from build123d import *

# Parameters (mm, degrees)
SKETCH_1_W           = 53
SKETCH_1_H           = 35
EXTRUDE_1_DEPTH      = 3.92
SKETCH_2_W           = 12
SKETCH_2_H           = 27
CUT_EXTRUDE_1_DEPTH  = 4
EXTRUDE_2_DEPTH      = 16.08
EXTRUDE_2_DEPTH_BACK = 3.92
SKETCH_3_W           = 12
SKETCH_3_H           = 7
SKETCH_4_W           = 12
SKETCH_4_H           = 3.92
EXTRUDE_3_DEPTH      = 8
SKETCH_5_R           = 2.86
CUT_EXTRUDE_2_DEPTH  = 37.889245045
EXTRUDE_4_DEPTH      = 4
SKETCH_8_W           = 53
SKETCH_8_H           = 3.92
EXTRUDE_5_DEPTH      = 20
FILLET_1_R           = 2.5
FILLET_2_R           = 11
FILLET_3_R           = 1
FILLET_4_R           = 2
SKETCH_9_W           = 20.08
SKETCH_9_H           = 8
CUT_EXTRUDE_5_DEPTH  = 67.886593574
SKETCH_6_R           = 6
CUT_EXTRUDE_3_DEPTH  = 6.5


with BuildPart() as part:
    # 스케치1 → 보스-돌출1 (new body)
    with BuildSketch(Plane.XY):
        Rectangle(SKETCH_1_W, SKETCH_1_H)
    extrude(amount=EXTRUDE_1_DEPTH)

    # 스케치2 → 컷-돌출1 (cut)
    with BuildSketch(Plane.XY.offset(3.92)):
        with Locations((-20.5, 4)):
            Rectangle(SKETCH_2_W, SKETCH_2_H)
        with Locations((20.5, 4)):
            Rectangle(SKETCH_2_W, SKETCH_2_H)
    extrude(amount=-CUT_EXTRUDE_1_DEPTH, mode=Mode.SUBTRACT)

    # 스케치3 → 보스-돌출2 (add, two sides: drawn at the far end of the back side and taken through both)
    with BuildSketch(Plane(origin=(0, 0, 0), x_dir=(-1, 0, 0), z_dir=(0, 0, -1)).offset(-EXTRUDE_2_DEPTH_BACK)):
        with Locations((-20.5, -6)):
            Rectangle(SKETCH_3_W, SKETCH_3_H)
        with Locations((20.5, -6)):
            Rectangle(SKETCH_3_W, SKETCH_3_H)
    extrude(amount=EXTRUDE_2_DEPTH + EXTRUDE_2_DEPTH_BACK)

    # 스케치4 → 보스-돌출3 (add)
    with BuildSketch(Plane.XZ.offset(9.5)):
        with Locations((-20.5, -14.12)):
            Rectangle(SKETCH_4_W, SKETCH_4_H)
        with Locations((20.5, -14.12)):
            Rectangle(SKETCH_4_W, SKETCH_4_H)
    extrude(amount=EXTRUDE_3_DEPTH)

    # 스케치5 → 컷-돌출2 (cut, through all)
    with BuildSketch(Plane(origin=(0, -2.5, 0), x_dir=(1, 0, 0), z_dir=(0, 1, 0))):
        with Locations(Location((-20.5, 6.08, 0), (0, 0, 180))):
            Circle(SKETCH_5_R)
        with Locations((20.5, 6.08)):
            Circle(SKETCH_5_R)
    extrude(amount=-CUT_EXTRUDE_2_DEPTH, mode=Mode.SUBTRACT)

    # 스케치7 → 보스-돌출4 (add)
    with BuildSketch(Plane.XY.offset(3.92)):
        Polygon((-14.5, -2.5), (-26.5, -2.5), (-26.5, -17.5), (26.5, -17.5), (26.5, -2.5), (14.5, -2.5), (14.5, 17.5), (-14.5, 17.5), align=None)
    extrude(amount=EXTRUDE_4_DEPTH)

    # 스케치8 → 보스-돌출5 (add)
    with BuildSketch(Plane.XZ.offset(17.5)):
        with Locations((0, 5.96)):
            Rectangle(SKETCH_8_W, SKETCH_8_H)
    extrude(amount=EXTRUDE_5_DEPTH)

    # 필렛1
    fillet_1_edges = [part.edges().sort_by_distance(p)[0] for p in [
        (14.5, -9.5, -6.08),
        (-14.5, -9.5, -6.08),
    ]]
    fillet(fillet_1_edges, radius=FILLET_1_R)

    # 필렛2
    fillet_2_edges = [part.edges().sort_by_distance(p)[0] for p in [
        (-14.5, 17.5, 3.96),
        (14.5, 17.5, 3.96),
    ]]
    fillet(fillet_2_edges, radius=FILLET_2_R)

    # 필렛3
    fillet_3_edges = [part.edges().sort_by_distance(p)[0] for p in [
        (26.5, -9.5, -6.08),
        (-26.5, -9.5, -6.08),
    ]]
    fillet(fillet_3_edges, radius=FILLET_3_R)

    # 필렛4
    fillet_4_edges = [part.edges().sort_by_distance(p)[0] for p in [
        (-20.5, -2.5, 7.92),
        (-26.5, -20, 7.92),
        (26.5, -20, 7.92),
        (20.5, -2.5, 7.92),
        (14.5, 2, 7.92),
        (0, -37.5, 7.92),
        (-14.5, 2, 7.92),
        (0, 17.5, 7.92),
        (-11.278174593, 14.278174593, 7.92),
        (11.278174593, 14.278174593, 7.92),
    ]]
    fillet(fillet_4_edges, radius=FILLET_4_R)

    # 스케치9 → 컷-돌출5 (cut, through all)
    with BuildSketch(Plane(origin=(26.5, 0, 0), x_dir=(0, 0, -1), z_dir=(1, 0, 0))):
        with Locations((6.04, -13.5)):
            Rectangle(SKETCH_9_W, SKETCH_9_H)
    extrude(amount=-CUT_EXTRUDE_5_DEPTH, mode=Mode.SUBTRACT)

    # 스케치6 → 컷-돌출3 (cut)
    with BuildSketch(Plane.XY):
        with Locations(Location((0, 2.5, 0), (0, 0, 180))):
            Circle(SKETCH_6_R)
    extrude(amount=CUT_EXTRUDE_3_DEPTH, mode=Mode.SUBTRACT)


solid = part.part
Verification items for the finished model (mm, model axes). A direction names the side the tool comes from. Round coordinates to 2 decimals unless told otherwise and drop trailing zeros. Loops run counter-clockwise (first coordinate to the right, second up) from the corner with the lowest first, then second, coordinate; pieces in that order, holes last. Notation, with made-up numbers: (73.25, -36) - (78.25, -36) arc R11 cw to (78.25, -32) - close; hole circle Ø1 at (-17.5, -31). An arc over 180 degrees is marked (long way). Use a Markdown table: item, result. Add a question column.
1. Section check A-A, the plane x = -20.5. Record the boundary of the cut face in (y, z), plus the area to 3 significant figures.
2. Release check for a two-part mould opening along X. For faces 4 (the face through (0.37, -36.9, 7.35)), 5 (the face through (14.5, 2, 3)), 6 (the face through (-14.5, -5, -8)), 7 (the face through (23.228, -5.951, -6.939)) record: released by +X, released by -X, zero draft, split by the parting line, or undercut.
3. Access from +Z, -Z, +X, -X, +Y, -Y to the whole of each face (thin tool, end or side, straight path). Record for faces 1 (the face through (0, -9.5, 1)), 2 (the face through (13.9, 1.08, 7.35)), 3 (the face through (-19.6, -3.07, 7.32)).
4. Section check D-D, the plane z = 1. Record the boundary of the cut face in (x, y).
5. Thickness scan on probe 1 along Y at (x, z) = (0, 2); probe 2 along Z at (x, y) = (20.5, -4.5); probe 3 along Z at (x, y) = (-9.5, 11). Record the ranges inside material, lowest first. Write a range as [from, to].
6. Section check B-B, the plane y = 2.5. Record the boundary of the cut face in (x, z), plus the area to 3 significant figures.
7. Gauge pin test, flat ends, axial feed: pin 1 (8.5 mm diameter, centred on x = -7, y = -26.5, fed in from -Z); pin 2 (6 mm diameter, centred on x = 20.5, z = -2.5, fed in from +Y); pin 3 (1.8 mm diameter, centred on y = 0, z = 3, fed in from -X). Record the tip position at first contact, or that the pin passes through.
8. Section check C-C, the plane z = -6.08. Record the boundary of the cut face in (x, y), plus the area to 3 significant figures.
Checks:
| question | item | result |
|---|---|---|
| 1 | outline | (-37.5, 4) - (-9.5, 4) - (-9.5, -3.22) - (-2.5, -3.22) - (-2.5, 5.92) arc R2 ccw to (-4.5, 7.92) - (-35.5, 7.92) arc R2 ccw to (-37.5, 5.92) - close; (-9.5, -16.08) - (-2.5, -16.08) - (-2.5, -8.94) - (-9.5, -8.94) - close |
| 1 | area | 236 mm^2 |
| 2 | face 4 | zero draft |
| 2 | face 5 | released by +X |
| 2 | face 6 | undercut |
| 2 | face 7 | undercut |
| 3 | face 1 | -Z, +X, -X, -Y |
| 3 | face 2 | +Z, +X, +Y |
| 3 | face 3 | +Z, -X, +Y |
| 4 | outline | (-26.5, -9.5) - (26.5, -9.5) - (26.5, -2.5) - (14.5, -2.5) - (14.5, 6.5) arc R11 ccw to (3.5, 17.5) - (-3.5, 17.5) arc R11 ccw to (-14.5, 6.5) - (-14.5, -2.5) - (-26.5, -2.5) - close; hole circle Ø12 at (0, 2.5) |
| 5 | probe 1 | y = [-9.5, -3.5], [8.5, 17.5] |
| 5 | probe 2 | z = [-16.08, -8.94], [-3.22, 7.92] |
| 5 | probe 3 | z = [0, 7.92] |
| 6 | outline | (-14.5, 0) - (-6, 0) - (-6, 6.5) - (6, 6.5) - (6, 0) - (14.5, 0) - (14.5, 5.92) arc R2 ccw to (12.5, 7.92) - (-12.5, 7.92) arc R2 ccw to (-14.5, 5.92) - close |
| 6 | area | 150 mm^2 |
| 7 | pin 1 | stops at z = 4 |
| 7 | pin 2 | stops at y = -2.5 |
| 7 | pin 3 | stops at x = -14.5 |
| 8 | outline | (-26.5, -8.5) arc R1 ccw to (-25.5, -9.5) - (-23.36, -9.5) - (-23.36, -2.5) - (-26.5, -2.5) - close; (-17.64, -9.5) - (-17, -9.5) arc R2.5 ccw to (-14.5, -7) - (-14.5, -2.5) - (-17.64, -2.5) - close; (14.5, -7) arc R2.5 ccw to (17, -9.5) - (17.64, -9.5) - (17.64, -2.5) - (14.5, -2.5) - close; (23.36, -9.5) - (25.5, -9.5) arc R1 ccw to (26.5, -8.5) - (26.5, -2.5) - (23.36, -2.5) - close |
| 8 | area | 84.8 mm^2 |
